from build123d import *

# Parameters (mm, degrees)
SKETCH1_W               = 22.86
SKETCH1_H               = 6.35
EXTRUDE1_DEPTH          = 50.8
EXTRUDE1_DEPTH_BACK     = 50.8
F_1_2_CLEARANCE_HOLE1_D = 13.49248
CUT_EXTRUDE1_DEPTH      = 7.35


with BuildPart() as part:
    # Sketch1 → Extrude1 (new body, two sides)
    with BuildSketch(Plane(origin=(0, 0, 0), x_dir=(0, 0, -1), z_dir=(1, 0, 0))) as extrude1_sk:
        Rectangle(SKETCH1_W, SKETCH1_H)
    extrude(amount=EXTRUDE1_DEPTH)
    extrude(extrude1_sk.sketch, amount=-EXTRUDE1_DEPTH_BACK)

    # 1_2 Clearance Hole1 (through all)
    with Locations(Plane(origin=(0, 3.175, 0), x_dir=(-1, 0, 0), z_dir=(0, 1, 0))):
        with Locations((31.75, -1.27), (-31.75, -1.27)):
            Hole(F_1_2_CLEARANCE_HOLE1_D / 2)

    # Sketch6 → Cut-Extrude1 (cut, through all)
    with BuildSketch(Plane(origin=(0, 3.175, 0), x_dir=(-1, 0, 0), z_dir=(0, 1, 0))):
        with BuildLine():
            Line((-9.452589884, -8.016875), (9.452589807, -8.016875))
            ThreePointArc((9.452589807, -8.016875), (16.199464807, -1.27), (9.452589807, 5.476875))
            Line((9.452589807, 5.476875), (-9.452589884, 5.476875))
            ThreePointArc((-9.452589884, 5.476875), (-16.199464884, -1.27), (-9.452589884, -8.016875))
        make_face()
    extrude(amount=-CUT_EXTRUDE1_DEPTH, mode=Mode.SUBTRACT)


solid = part.part
Work out the finished part from the listing and answer in its coordinate system (mm). A direction names the side the tool comes from. Give positions to 0.01 mm unless a question says otherwise; leave off trailing zeros. Write each loop counter-clockwise with the first axis right and the second up, starting at its lowest first coordinate (ties: lowest second). Pieces come first, ordered by that corner, then holes. Notation, with made-up numbers: (45.25, 86.25) - (59.25, 86.25) arc R26 ccw to (59.25, 121.25) - close; hole circle Ø9 at (14.25, -28.5). An arc over 180 degrees is marked (long way). One line per item, written item: value. Start each with the question number.
1. Find section D-D (x = 0). Write down the section's boundary in (y, z) (3 decimals), then the cut area to 3 significant figures.
2. Find section C-C (z = -1.27). Write down the section's boundary in (x, y) (3 decimals).
3. Given pin 1 (6 mm diameter, centred on x = 1, z = -5.5, fed in from -Y) (3 decimals); pin 2 (11 mm diameter, centred on x = 31.75, z = -1.27, fed in from +Y), each flat-ended and moving along its own axis, determine where each tip first touches the part or whether it passes through.
4. Find section B-B (x = -31.75). Write down the section's boundary in (y, z) (3 decimals).
5. Find section A-A (y = -0.5). Write down the section's boundary in (x, z), then the cut area to 3 significant figures.
6. For faces 1 (the flat face through (1, 0, -11.43)), 2 (the flat face through (0, 0, 5.477)), determine the directions among +Z, -Z, +X, -X, +Y, -Y from which every point of the face is accessible in a straight line to the end or side of a thin tool.
7. Consider probe 1 along Z at (x, y) = (31.75, 0.75); probe 2 along X at (y, z) = (-2.5, -2.5); probe 3 along X at (y, z) = (2, 2.5). Determine where each line is inside the solid, lowest interval first.
8. For a pull along Z with two mould halves and no side action, classify faces 3 (the cylindrical face through (25.01, -0.04, -0.97)), 4 (the flat face through (1, 0, 11.43)), 5 (the flat face through (0, 0, -8.017)), 6 (the flat face through (50.8, 0, 0)) as +Z half, -Z half, draft (parallel to the pull), parting line (faces both ways), or undercut.
Geometry results:
1. outline: (-3.175, -11.43) - (3.175, -11.43) - (3.175, -8.017) - (-3.175, -8.017) - close; (-3.175, 5.477) - (3.175, 5.477) - (3.175, 11.43) - (-3.175, 11.43) - close
1. area: 59.5 mm2
2. outline: (-50.8, -3.175) - (-38.496, -3.175) - (-38.496, 3.175) - (-50.8, 3.175) - close; (-25.004, -3.175) - (-16.199, -3.175) - (-16.199, 3.175) - (-25.004, 3.175) - close; (16.199, -3.175) - (25.004, -3.175) - (25.004, 3.175) - (16.199, 3.175) - close; (38.496, -3.175) - (50.8, -3.175) - (50.8, 3.175) - (38.496, 3.175) - close
3. pin 1: y = -3.175
3. pin 2: through
4. outline: (-3.175, -11.43) - (3.175, -11.43) - (3.175, -8.016) - (-3.175, -8.016) - close; (-3.175, 5.476) - (3.175, 5.476) - (3.175, 11.43) - (-3.175, 11.43) - close
5. outline: (-50.8, -11.43) - (50.8, -11.43) - (50.8, 11.43) - (-50.8, 11.43) - close; hole circle Ø13.49 at (-31.75, -1.27); hole (-9.45, -8.02) - (9.45, -8.02) arc R6.75 ccw to (9.45, 5.48) - (-9.45, 5.48) arc R6.75 ccw to start; hole circle Ø13.49 at (31.75, -1.27)
5. area: 1,640 mm2
6. face 1: -Z, +X, -X, +Y, -Y
6. face 2: +Y, -Y
7. probe 1: -11.43 to -8.02, 5.48 to 11.43
7. probe 2: -50.8 to -38.38, -25.12 to -16.09, 16.09 to 25.12, 38.38 to 50.8
7. probe 3: -50.8 to -37.34, -26.16 to -15.05, 15.05 to 26.16, 37.34 to 50.8
8. face 3: undercut
8. face 4: +Z half
8. face 5: undercut
8. face 6: draft
